Work out the finished part from the listing and answer in its coordinate system (mm). A direction names the side the tool comes from. Round coordinates to 2 decimals unless told otherwise and drop trailing zeros. Order: outer loops, then holes, each group sorted by start corner. A loop starts at its lowest first (then second) coordinate and runs counter-clockwise, first axis right, second up. Notation, with made-up numbers: (4.5, 10) - (12.5, 10) arc R21 cw to (12.5, 31) - close; hole circle Ø6 at (21, 30.5). An arc over 180 degrees is marked (long way). Use CSV: the item, a comma, the result in double quotes.
from build123d import *

# Parameters (mm, degrees)
SKETCH1_R               = 19.05
EXTRUDE1_DEPTH          = 31.75
EXTRUDE1_DEPTH_BACK     = 31.75
SKETCH2_R               = 15.875
CUT_EXTRUDE1_DEPTH      = 32.75
CUT_EXTRUDE1_DEPTH_BACK = 32.75
SKETCH3_R               = 21.59
SKETCH3_R_2             = 19.05
EXTRUDE_THIN1_DEPTH     = 1.27
LPATTERN1_COUNT         = 11
LPATTERN1_PITCH         = 2.54
LPATTERN1_COL_COUNT     = 10
LPATTERN1_COL_PITCH     = 2.54


with BuildPart() as part:
    # Sketch1 → Extrude1 (new body, two sides)
    with BuildSketch(Plane(origin=(0, 0, 0), x_dir=(1, 0, 0), z_dir=(0, 1, 0))) as extrude1_sk:
        Circle(SKETCH1_R)
    extrude(amount=EXTRUDE1_DEPTH)
    extrude(extrude1_sk.sketch, amount=-EXTRUDE1_DEPTH_BACK)

    # Sketch2 → Cut-Extrude1 (cut, two sides)
    with BuildSketch(Plane(origin=(0, 0, 0), x_dir=(1, 0, 0), z_dir=(0, 1, 0))) as cut_extrude1_sk:
        Circle(SKETCH2_R)
    extrude(amount=CUT_EXTRUDE1_DEPTH, mode=Mode.SUBTRACT)
    extrude(cut_extrude1_sk.sketch, amount=-CUT_EXTRUDE1_DEPTH_BACK, mode=Mode.SUBTRACT)

    # Sketch3 → Extrude-Thin1 (add)
    with BuildSketch(Plane(origin=(0, 0, 0), x_dir=(1, 0, 0), z_dir=(0, 1, 0))):
        Circle(SKETCH3_R)
        Circle(SKETCH3_R_2, mode=Mode.SUBTRACT)
    extrude_thin1 = extrude(amount=EXTRUDE_THIN1_DEPTH)

    # LPattern1: Extrude-Thin1 ×11
    with Locations(*[(0, -i * LPATTERN1_PITCH, 0) for i in range(1, LPATTERN1_COUNT)]):
        add(extrude_thin1)

    # LPattern1 col: Extrude-Thin1 ×10
    with Locations(*[(0, i * LPATTERN1_COL_PITCH, 0) for i in range(1, LPATTERN1_COL_COUNT)]):
        add(extrude_thin1)


solid = part.part
(1) Find the intervals of material crossed by L1, parallel to X at y = 10.5, z = 0 (3 decimals); L2, parallel to Z at x = 0, y = 7 (3 decimals), in increasing order. Write a range as from..to.
Findings below:
L1,"x = -21.59..-15.875, 15.875..21.59"
L2,"z = -19.05..-15.875, 15.875..19.05"
(2) The mould has two halves that part along Y. Classify faces 1 (the flat face through (7.9, 20.32, 17.5)), 2 (the cylindrical face through (-15.913, -4.454, -14.592)), 3 (the flat face through (7.9, 24.13, 17.5)): released by +Y, released by -Y, zero draft, split by the parting line, or undercut.
Findings below:
face 1,"undercut"
face 2,"zero draft"
face 3,"released by +Y"
(3) Find section A-A (y = 26). Determine the outline of the cut face in (x, z) (3 decimals), and give its area (3 significant figures).
Findings below:
outline,"circle Ø38.1 at (0, 0); hole circle Ø31.75 at (0, 0)"
area,"348 mm²"
(4) Each of these flat-tipped pins is pushed along its axis until it touches: pin 1 (1 mm diameter, centred on x = 14.5, y = -19, fed in from -Z); pin 2 (6 mm diameter, centred on x = 8.5, y = -15, fed in from +Z); pin 3 (6 mm diameter, centred on y = 11.5, z = 14, fed in from -X). Where does it stop, or does it pass through?
Findings below:
pin 1,"stops at z = -16.43"
pin 2,"stops at z = 20.88"
pin 3,"stops at x = -18.58"
(5) For faces 4 (the flat face through (7.9, -15.24, 17.5)), 5 (the cylindrical face through (-15.913, 10.786, -14.592)), determine the directions among +Z, -Z, +X, -X, +Y, -Y from which every point of the face is accessible in a straight line to the end or side of a thin tool.
Findings below:
face 4,"none"
face 5,"+Y, -Y"
